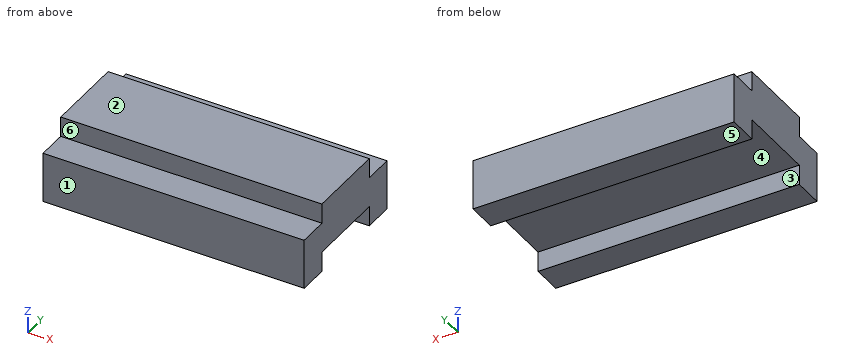
```python
from build123d import *

# Parameters (mm, degrees)
F0_W     = 88.9
F0_H     = 44.45
F1_DEPTH = 165.1
F2_W     = 19.05
F2_H     = 12.7
F2_W_2   = 50.8
F3_DEPTH = 165.1


with BuildPart() as f1:
    # F0 (on Right) → F1 (new body)
    with BuildSketch(Plane.YZ):
        Rectangle(F0_W, F0_H)
    extrude(amount=F1_DEPTH)

    # F2 (on face) → F3 (cut)
    with BuildSketch(Plane.YZ.offset(165.1)):
        with Locations((-34.925, 15.875)):
            Rectangle(F2_W, F2_H)
        with Locations((34.925, 15.875)):
            Rectangle(F2_W, F2_H)
        with Locations((0, -15.875)):
            Rectangle(F2_W_2, F2_H)
    extrude(amount=-F3_DEPTH, mode=Mode.SUBTRACT)


solid = f1.part
```
CAD build for the part. Positions are in the model's coordinates, mm. Face numbers are marked on the shaded views. A direction names the side the tool comes from. Round coordinates to 2 decimals unless told otherwise and drop trailing zeros. Order: outer loops, then holes, each group sorted by start corner. A loop starts at its lowest first (then second) coordinate and runs counter-clockwise, first axis right, second up.
Q1. Which spindle directions (+Z, -Z, +X, -X, +Y, -Y) get a long thin tool onto all of the face, cutting with end or side? Do the marked faces 5 and 6. Say none if no direction does.
Q2. Slice it at A-A (z = -11.5). Write the cut outline in (x, y), and give its area (3 significant figures).
Q3. Slice it at B-B (x = 20). Write the cut outline in (y, z) (3 decimals), and give its area (3 significant figures).
Q4. Slice it at D-D (z = 14). Write the cut outline in (x, y).
Q5. Drop flat-ended pins along their axis: pin 1 (4 mm diameter, centred on x = 59, z = 14.5, fed in from -Y); pin 2 (6.5 mm diameter, centred on x = 122.5, z = 17.5, fed in from +Y); pin 3 (9.5 mm diameter, centred on x = 104, y = 31, fed in from +Z) (3 decimals). Give the stop position or say it passes through.
Q6. Wall check: L1, parallel to Y at x = 46, z = -13.5; L2, parallel to Z at x = 68.5, y = -27.5 (3 decimals); L3, parallel to Y at x = 24, z = 19. Give the ranges that are in metal, low to high.
Q7. Two-plate mould, pull along Y, no slides. Class the marked faces 1, 2, 3 and 4: pulls with the +Y half, pulls with the -Y half, needs draft (parallel to the pull), parting line crosses it, or undercut.
Q8. Slice it at C-C (y = -8). Write the cut outline in (x, z) (3 decimals), and give its area (3 significant figures).
Results below:
1. face 5: -Z, +X, -X, +Y, -Y
1. face 6: +Z, +X, -X, -Y
2. outline: (0, -44.45) - (165.1, -44.45) - (165.1, -25.4) - (0, -25.4) - close; (0, 25.4) - (165.1, 25.4) - (165.1, 44.45) - (0, 44.45) - close
2. area: 6,290 mm2
3. outline: (-44.45, -22.225) - (-25.4, -22.225) - (-25.4, -9.525) - (25.4, -9.525) - (25.4, -22.225) - (44.45, -22.225) - (44.45, 9.525) - (25.4, 9.525) - (25.4, 22.225) - (-25.4, 22.225) - (-25.4, 9.525) - (-44.45, 9.525) - close
3. area: 2,820 mm2
4. outline: (0, -25.4) - (165.1, -25.4) - (165.1, 25.4) - (0, 25.4) - close
5. pin 1: stops at y = -25.4
5. pin 2: stops at y = 25.4
5. pin 3: stops at z = 9.525
6. L1: y = -44.45 to -25.4, 25.4 to 44.45
6. L2: z = -22.225 to 9.525
6. L3: y = -25.4 to 25.4
7. face 1: pulls with the -Y half
7. face 2: needs draft
7. face 3: undercut
7. face 4: undercut
8. outline: (0, -9.525) - (165.1, -9.525) - (165.1, 22.225) - (0, 22.225) - close
8. area: 5,240 mm2
